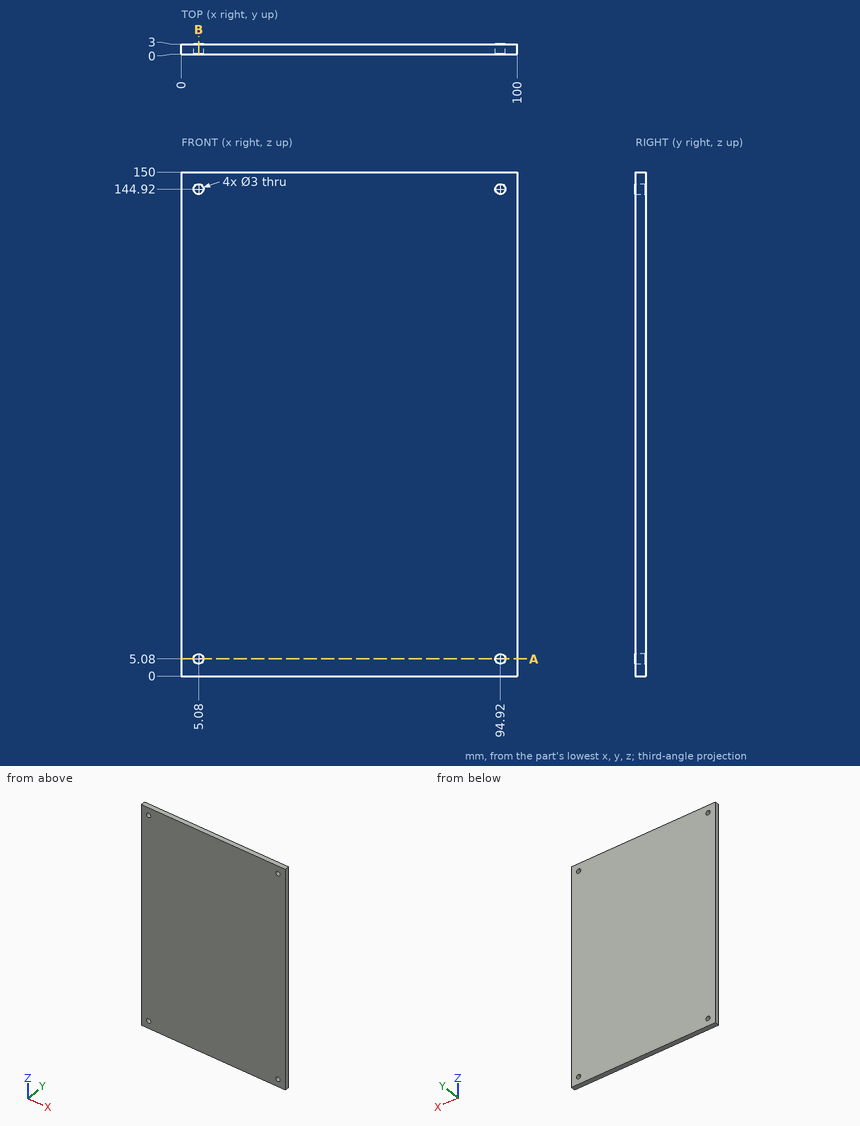
The drawing under review shows one solid part. Ordinate dimensions are in mm from its lowest x, y, z. Give positions to 0.01 mm unless a question says otherwise; leave off trailing zeros. Order: outer loops, then holes, each group sorted by start corner. A loop starts at its lowest first (then second) coordinate and runs counter-clockwise, first axis right, second up. Notation, with made-up numbers: (-4, -37.5) -> (18, -37.5) arc R32 cw to (18, -4.5) -> close; hole circle Ø7 at (3, 59.5). An arc over 180 degrees is marked (long way). Write item = value, one per line.
1) We need section B-B, the plane x = 5.08. Give the boundary of the cut face in (y, z), and give its area (3 significant figures).
Findings:
outline = (0, 0) -> (3, 0) -> (3, 3.58) -> (0, 3.58) -> close; (0, 6.58) -> (3, 6.58) -> (3, 143.42) -> (0, 143.42) -> close; (0, 146.42) -> (3, 146.42) -> (3, 150) -> (0, 150) -> close
area = 432 mm^2
2) Insertion check: pin 1 (3.5 mm diameter, centred on x = 5.08, z = 5.08, fed in from +Y). The pin has a flat end and moves straight along its axis. Give the tip position at first contact, or say it passes through.
Findings:
pin_1 = 3
3) We need section A-A, the plane z = 5.08. Give the boundary of the cut face in (x, y).
Findings:
outline = (0, 0) -> (3.58, 0) -> (3.58, 3) -> (0, 3) -> close; (6.58, 0) -> (93.42, 0) -> (93.42, 3) -> (6.58, 3) -> close; (96.42, 0) -> (100, 0) -> (100, 3) -> (96.42, 3) -> close
4) To check wall thickness, follow L1, parallel to X at y = 1.1, z = 144.92; L2, parallel to Z at x = 94.92, y = 1.9. State the ranges of each line that lie inside material, in increasing order. Write a range as from..to.
Findings:
L1 = 0..3.58, 6.58..93.42, 96.42..100
L2 = 0..3.58, 6.58..143.42, 146.42..150
